Geometry check sheet. Reference: drawing and pictorial views, mm from the part's lowest x, y, z. Give positions to 0.01 mm unless a question says otherwise; leave off trailing zeros. Write each loop counter-clockwise with the first axis right and the second up, starting at its lowest first coordinate (ties: lowest second). Pieces come first, ordered by that corner, then holes. Notation, with made-up numbers: (47, 58) -> (62, 58) arc R32 cw to (62, 97) -> close; hole circle Ø3 at (56.5, -38.75). An arc over 180 degrees is marked (long way). Use a Markdown table: item, result. Add a question column.
1. Cross-section at A-A (z = 8). Enter the section's corners in (x, y), then the cut area to 3 significant figures.
2. Cross-section at C-C (y = 6.75). Enter the section's corners in (x, z).
3. Scan lines: probe 1 along X at (y, z) = (1, 29); probe 2 along Z at (x, y) = (43, 0.5); probe 3 along Z at (x, y) = (44, 5). Record each from-to range of solid material in increasing order. Write a range as [from, to].
4. Release check for a two-part mould opening along X. For the marked faces 1, 2 and 3 record: released by +X, released by -X, zero draft, split by the parting line, or undercut.
5. Cross-section at B-B (z = 30). Enter the section's corners in (x, y).
6. Gauge pin test, flat end, axial feed: P1, Ø5.5, axis at x = 20, z = 30, coming from the +Y side. Record the tip position at first contact, or that the pin passes through.
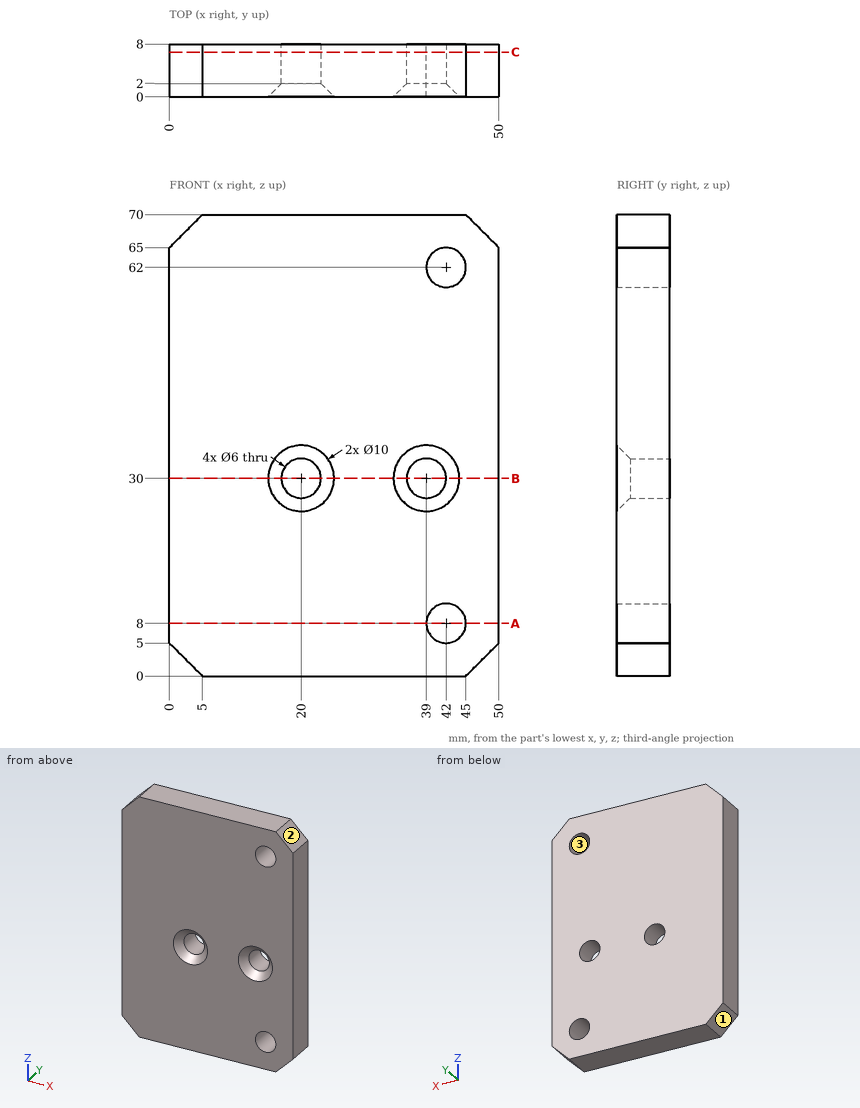
Worked answers:
| question | item | result |
|---|---|---|
| 1 | outline | (0, 0) -> (39, 0) -> (39, 8) -> (0, 8) -> close; (45, 0) -> (50, 0) -> (50, 8) -> (45, 8) -> close |
| 1 | area | 352 mm² |
| 2 | outline | (0, 5) -> (5, 0) -> (45, 0) -> (50, 5) -> (50, 65) -> (45, 70) -> (5, 70) -> (0, 65) -> close; hole circle Ø6 at (20, 30); hole circle Ø6 at (39, 30); hole circle Ø6 at (42, 8); hole circle Ø6 at (42, 62) |
| 3 | probe 1 | x = [0, 16.13], [23.87, 35.13], [42.87, 50] |
| 3 | probe 2 | z = [0, 5.17], [10.83, 27.94], [32.06, 59.17], [64.83, 70] |
| 3 | probe 3 | z = [0, 5.76], [10.24, 59.76], [64.24, 70] |
| 4 | face 1 | released by -X |
| 4 | face 2 | released by +X |
| 4 | face 3 | undercut |
| 5 | outline | (0, 0) -> (15, 0) -> (17, 2) -> (17, 8) -> (0, 8) -> close; (23, 2) -> (25, 0) -> (34, 0) -> (36, 2) -> (36, 8) -> (23, 8) -> close; (42, 2) -> (44, 0) -> (50, 0) -> (50, 8) -> (42, 8) -> close |
| 6 | P1 | passes through |
